Autodesk Inventor part; units mm, degrees
ref_plane "YZ Plane" through (0, 0, 0) normal (1, 0, 0) x (0, 1, 0)
ref_plane "XZ Plane" through (0, 0, 0) normal (0, 1, 0) x (-1, 0, 0)
ref_plane "XY Plane" through (0, 0, 0) normal (0, 0, 1) x (1, 0, 0)
sketch "Base" plane through (0, 0, 0) normal (0, 0, 1) x (1, 0, 0)
  line L0 (0, 0) -> (0, -15) construction
  line L1 (0, -15) -> (2, -15)
  line L2 (2, -15) -> (4, -13.0641)
  line L3 (5, -3.4641) -> (3, 0)
  line L4 (3, 0) -> (0, 0)
  line L5 (4, -13.0641) -> (5, -3.4641)
  line L6 (0, -15) -> (0.7289, -11.25)
  line L7 (0.7289, -11.25) -> (0, 0)
  dimension "d0" = 15
  dimension "d1" = 3
  dimension "d2" = 2
  dimension "d3" = 5
  dimension "d8" = 4
  dimension "d12" = 120
  dimension "d14" = 9.6
  dimension "d23" = 11.25
  dimension "d24" = 79
extrude "BaseFeature" add sketch "Base" along normal blind 9
sketch "TopProfile" plane through (0.7289, -11.25, 0) normal (-0.9979, -0.0647, 0) x (0, 0, 1)
  line L0 (0, 7.4934) -> (9, 7.4934)
  line L1 (2, 11.2736) -> (7, 11.2736)
  line L2 (7, 11.2736) -> (9, 7.4934)
  line L3 (9, 7.4934) -> (6.5, -3.8243)
  line L4 (6.5, -3.8243) -> (2.5, -3.8243)
  line L5 (2.5, -3.8243) -> (0, 7.4934)
  line L6 (0, 7.4934) -> (2, 11.2736)
  line L7 (0, 11.2736) -> (9, 11.2736)
  line L8 (0, -3.8243) -> (9, -3.8243)
  point P0 (4.5, 11.2736)
  point P1 (4.5, -3.8243)
  dimension "d27" = 5
  dimension "d28" = 4
extrude "TopProfileFeature" cut sketch "TopProfile" along normal through all both and the other way through all keep common part
equation "\"d14\" = 0.64 * d0"
equation "\"d23\" = 0.75 * d0"
properties part number "DistalPhalangeIndexMiddle"
Source: CAD feature listing. Evaluate the final solid. Frame: model axes, mm. Round coordinates to 2 decimals unless told otherwise and drop trailing zeros. Loops run counter-clockwise (first coordinate to the right, second up) from the corner with the lowest first, then second, coordinate; pieces in that order, holes last.
Q1. Mould query, pull axis Y, two halves, no side actions, for faces 1 (the face through (0.37, -5.7, 4.44)), 2 (the face through (4.493, -8.331, 4.437)), 3 (the face through (0.36, -13.15, 4.46)), 4 (the face through (2, 0, 4)). Classes: pulls with the +Y half, pulls with the -Y half, needs draft (parallel to the pull), parting line crosses it, or undercut.
Q2. Section C-C, the plane y = -3.25. Return loops of the section in (x, z).
Q3. Ray query, line 1 (Z direction, x = 3.65, y = -1.5); line 2 (Z direction, x = 2.7, y = -8); line 3 (X direction, y = -2.75, z = 3.75). Return the intervals inside material, ascending.
Q4. Section B-B, the plane x = 0.95. Return loops of the section in (y, z).
Q5. First-contact query: P1, Ø1.5, axis at y = -2.5, z = 6, coming from the -X side; P2, Ø3, axis at x = 2.5, y = -8, coming from the +Z side; P3, Ø1.5, axis at y = -1.5, z = 5.5, coming from the +X side. Flat tips, straight axial feed; report the tip coordinate or a pass-through.
Q6. Section D-D, the plane x = 2.7. Return loops of the section in (y, z).
Solutions:
1. face 1: undercut
1. face 2: pulls with the -Y half
1. face 3: undercut
1. face 4: pulls with the +Y half
2. outline: (0.21, 0.28) - (4.88, 0.12) - (4.88, 8.88) - (0.21, 8.72) - close
3. line 1: z = 1.08 to 7.92
3. line 2: z = 0.97 to 8.03
3. line 3: x = 0.18 to 4.59
4. outline: (-15, 2.49) - (-3.73, 0) - (0, 1.97) - (0, 7.03) - (-3.73, 9) - (-15, 6.51) - close
5. P1: stops at x = 0.11
5. P2: stops at z = 8.37
5. P3: stops at x = 4.3
6. outline: (-14.32, 2.36) - (-3.61, 0) - (0, 1.91) - (0, 7.09) - (-3.61, 9) - (-14.32, 6.64) - close
